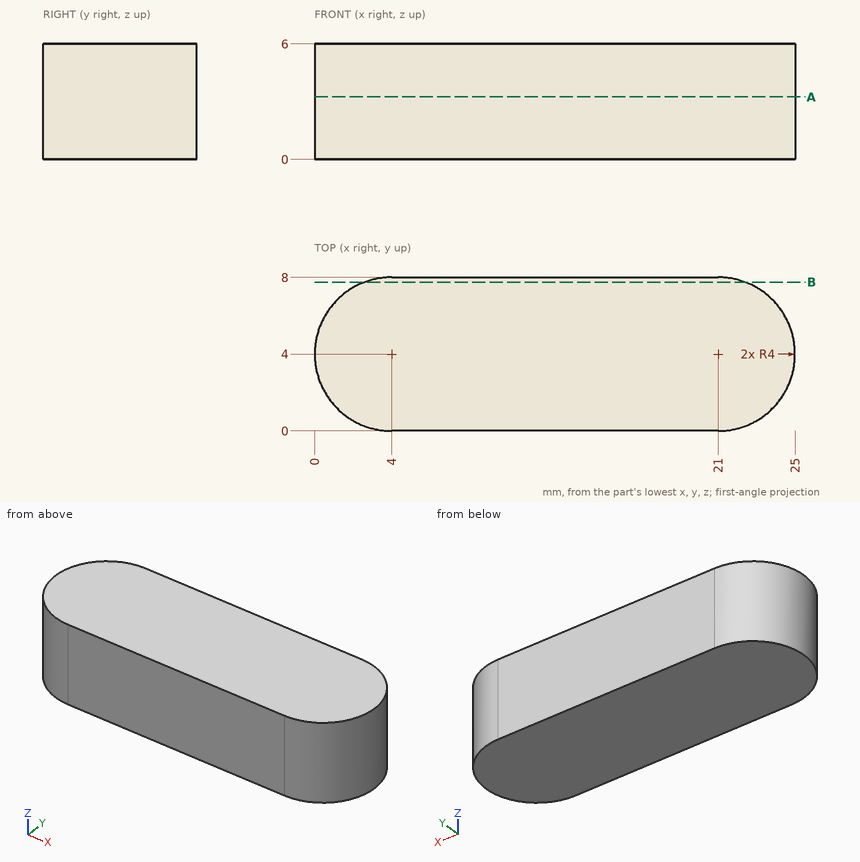
Can you work these out from the drawing? Everything is in mm from the part's minimum corner. Give positions to 0.01 mm unless a question says otherwise; leave off trailing zeros. Loops run counter-clockwise (first coordinate to the right, second up) from the corner with the lowest first, then second, coordinate; pieces in that order, holes last. Notation, with made-up numbers: M -18.5,24 L -7.5,24 A20 cw -7.5,44 Z; hole C 45.5,0.5 d10. An arc over 180 degrees is marked long. Use CSV: the item, a comma, the result in double quotes. Start each with the question number.
1. If I drill on L1, parallel to X at y = 5, z = 4.35; L2, parallel to X at y = 7.25, z = 5.5; L3, parallel to Y at x = 1.5, z = 1.6, over which ranges is the centre line in solid material (lowest first)?
2. For P1, Ø1, axis at y = 1, z = 2.5, coming from the +X side, with a flat end and sliding along its axis, tell me the tip position at first contact or that it passes through.
3. Imagine slicing it at B-B, the plane y = 7.75. Write out the boundary of the cut face in (x, z), plus the area to 3 significant figures.
4. Imagine slicing it at A-A, the plane z = 3.25. Write out the boundary of the cut face in (x, y), plus the area to 3 significant figures.
Response values:
1,L1,"0.13 to 24.87"
1,L2,"1.67 to 23.33"
1,L3,"0.88 to 7.12"
2,P1,"x = 24.12"
3,outline,"M 2.61,0 L 22.39,0 L 22.39,6 L 2.61,6 Z"
3,area,"119 mm^2"
4,outline,"M 4,0 L 21,0 A4 ccw 21,8 L 4,8 A4 ccw Z"
4,area,"186 mm^2"
